Could you check a few things on this model? Use its own coordinates, in mm. Face numbers are marked on the shaded views. Round coordinates to 2 decimals unless told otherwise and drop trailing zeros. Loops run counter-clockwise (first coordinate to the right, second up) from the corner with the lowest first, then second, coordinate; pieces in that order, holes last. Notation, with made-up numbers: (37.25, 69.25) - (68.25, 69.25) arc R31 cw to (68.25, 96.25) - close; hole circle Ø1 at (-32.5, 40). An arc over 180 degrees is marked (long way). Answer as CSV lines item,"result". Start each with the question number.
1) Please list where these lines run through material, in increasing order: line 1 along Z through (x, y) = (5.5, 2.25); line 2 along Z through (x, y) = (4, 2.75); line 3 along X through (y, z) = (2, 77.5).
2) Suppose I cut it at B-B, the plane z = 93. Write out the boundary of the cut face in (x, y), then the cut area to 3 significant figures.
3) Suppose I cut it at A-A, the plane z = 137. Write out the boundary of the cut face in (x, y), then the cut area to 3 significant figures.
4) I'm going to push flat-ended pins straight in: pin 1 Ø3 at (x, z) = (0.5, 89) entering from -Y; pin 2 Ø5 at (x, z) = (0.5, 129.5) entering from +Y; pin 3 Ø1 at (x, z) = (-3, 51.5) entering from -Y. Where does each tip first touch, or does it pass through?
5) We'd pull the mould along Z, two halves only. Please class the marked faces 1, 2 and 3: pulls with the +Z half, pulls with the -Z half, needs draft (parallel to the pull), parting line crosses it, or undercut.
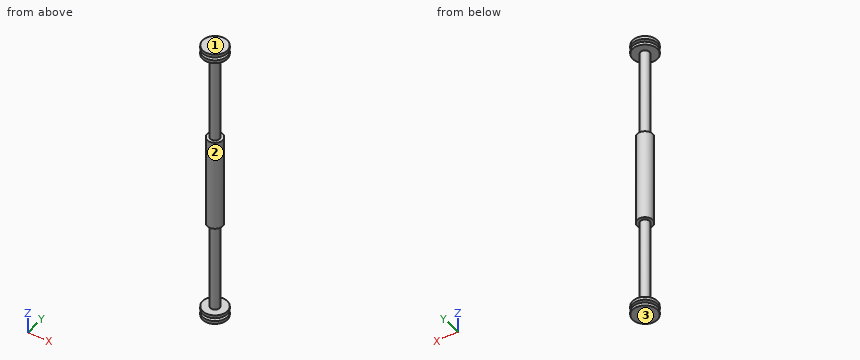
```python
from build123d import *

# Parameters (mm, degrees)
SKETCH_1_R       = 3
EXTRUDE_1_DEPTH  = 180
SKETCH_2_R       = 8
EXTRUDE_2_DEPTH  = 2
EXTRUDE_START    = -178
SKETCH_2_2_R     = 8
EXTRUDE_3_DEPTH  = 2
EXTRUDE_START_2  = -2
SKETCH_1_2_R     = 3
EXTRUDE_4_DEPTH  = 2
EXTRUDE_START_3  = 180
SKETCH_1_3_R     = 3
EXTRUDE_5_DEPTH  = 2
EXTRUDE_START_4  = 4
SKETCH_2_3_R     = 8
EXTRUDE_6_DEPTH  = 2
EXTRUDE_START_5  = -182
SKETCH_2_4_R     = 8
EXTRUDE_7_DEPTH  = 2
EXTRUDE_START_6  = -64
SKETCH_3_R       = 5
EXTRUDE_10_DEPTH = 60


with BuildPart() as part:
    # 草图1 → 凸台-拉伸1 (new body)
    with BuildSketch(Plane.XY):
        with Locations(Location((0, 0, 0), (0, 0, 180))):
            Circle(SKETCH_1_R)
    extrude(amount=EXTRUDE_1_DEPTH)

    # 草图2 → 凸台-拉伸2 (add)
    with BuildSketch(Plane.XY.offset(180)):
        Circle(SKETCH_2_R)
    extrude(amount=-EXTRUDE_2_DEPTH)

    # 草图2<2> → 凸台-拉伸3 (add)
    with BuildSketch(Plane.XY.offset(180).offset(EXTRUDE_START)):
        Circle(SKETCH_2_2_R)
    extrude(amount=-EXTRUDE_3_DEPTH)

    # 草图1<2> → 凸台-拉伸4 (add)
    with BuildSketch(Plane.XY.offset(EXTRUDE_START_2)):
        with Locations(Location((0, 0, 0), (0, 0, 180))):
            Circle(SKETCH_1_2_R)
    extrude(amount=EXTRUDE_4_DEPTH)

    # 草图1<3> → 凸台-拉伸5 (add)
    with BuildSketch(Plane.XY.offset(EXTRUDE_START_3)):
        with Locations(Location((0, 0, 0), (0, 0, 180))):
            Circle(SKETCH_1_3_R)
    extrude(amount=EXTRUDE_5_DEPTH)

    # 草图2<3> → 凸台-拉伸6 (add)
    with BuildSketch(Plane.XY.offset(180).offset(EXTRUDE_START_4)):
        Circle(SKETCH_2_3_R)
    extrude(amount=-EXTRUDE_6_DEPTH)

    # 草图2<4> → 凸台-拉伸7 (add)
    with BuildSketch(Plane.XY.offset(180).offset(EXTRUDE_START_5)):
        Circle(SKETCH_2_4_R)
    extrude(amount=-EXTRUDE_7_DEPTH)

    # 草图3 → 凸台-拉伸10 (add)
    with BuildSketch(Plane.XY.offset(184).offset(EXTRUDE_START_6)):
        Circle(SKETCH_3_R)
    extrude(amount=-EXTRUDE_10_DEPTH)


solid = part.part
```
Filled sheet:
1,line 1,"-4 to -2, 0 to 2, 178 to 180, 182 to 184"
1,line 2,"-4 to -2, 0 to 2, 60 to 120, 178 to 180, 182 to 184"
1,line 3,"-4.58 to 4.58"
2,outline,"circle Ø10 at (0, 0)"
2,area,"78.5 mm²"
3,outline,"circle Ø6 at (0, 0)"
3,area,"28.3 mm²"
4,pin 1,"y = -5"
4,pin 2,"y = 3"
4,pin 3,"y = -1.66"
5,face 1,"pulls with the +Z half"
5,face 2,"undercut"
5,face 3,"pulls with the -Z half"
